Build history of the part. All positions in model axes, mm. Give positions to 0.01 mm unless a question says otherwise; leave off trailing zeros. Order: outer loops, then holes, each group sorted by start corner. A loop starts at its lowest first (then second) coordinate and runs counter-clockwise, first axis right, second up. Notation, with made-up numbers: (14.5, 36) - (20.5, 36) arc R22 ccw to (20.5, 45) - close; hole circle Ø10 at (-21.5, 48). An arc over 180 degrees is marked (long way). One line per item, written item: value.
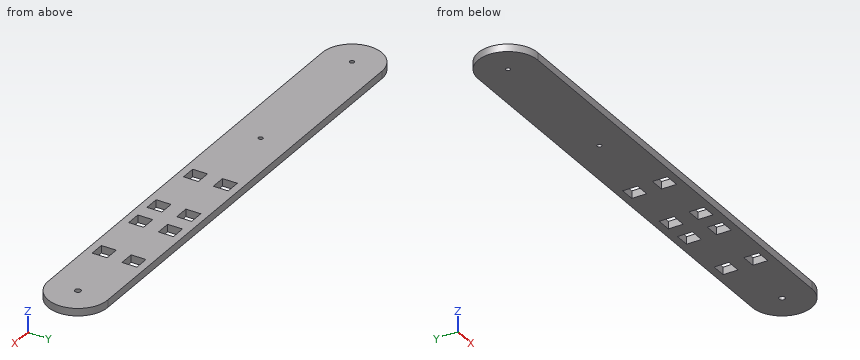
```python
from build123d import *

# Parameters (mm, degrees)
SKETCH1_R           = 1.5
SKETCH1_R_2         = 2
SKETCH1_W           = 10
SKETCH1_H           = 10
BOSS_EXTRUDE1_DEPTH = 5


with BuildPart() as part:
    # Sketch1 → Boss-Extrude1 (new body)
    with BuildSketch(Plane.XY):
        with BuildLine():
            Line((-126.904376013, 20), (173.095623987, 20))
            ThreePointArc((173.095623987, 20), (193.095623987, 0), (173.095623987, -20))
            Line((173.095623987, -20), (-126.904376013, -20))
            ThreePointArc((-126.904376013, -20), (-146.904376013, 0), (-126.904376013, 20))
        make_face()
        with Locations((-126.904376013, 0)):
            Circle(SKETCH1_R, mode=Mode.SUBTRACT)
        with Locations((173.095623987, 0)):
            Circle(SKETCH1_R_2, mode=Mode.SUBTRACT)
        with Locations((-26.904376013, 0)):
            Circle(SKETCH1_R, mode=Mode.SUBTRACT)
        Polygon((63.095623987, 15), (73.095623987, 15), (73.095623987, 10), (73.095623987, 5), (63.095623987, 5), (63.095623987, 10), align=None, mode=Mode.SUBTRACT)
        Polygon((83.095623987, 10), (83.095623987, 5), (93.095623987, 5), (93.095623987, 10), (93.095623987, 15), (83.095623987, 15), align=None, mode=Mode.SUBTRACT)
        Polygon((123.095623987, 10), (123.095623987, 5), (133.095623987, 5), (133.095623987, 10), (133.095623987, 15), (123.095623987, 15), align=None, mode=Mode.SUBTRACT)
        Polygon((33.095623987, -15), (23.095623987, -15), (23.095623987, -10), (23.095623987, -5), (33.095623987, -5), (33.095623987, -10), align=None, mode=Mode.SUBTRACT)
        Polygon((63.095623987, -15), (73.095623987, -15), (73.095623987, -10), (73.095623987, -5), (63.095623987, -5), (63.095623987, -10), align=None, mode=Mode.SUBTRACT)
        Polygon((83.095623987, -10), (83.095623987, -5), (93.095623987, -5), (93.095623987, -10), (93.095623987, -15), (83.095623987, -15), align=None, mode=Mode.SUBTRACT)
        Polygon((123.095623987, -5), (133.095623987, -5), (133.095623987, -10), (133.095623987, -15), (123.095623987, -15), (123.095623987, -10), align=None, mode=Mode.SUBTRACT)
        with Locations((28.095623987, 10)):
            Rectangle(SKETCH1_W, SKETCH1_H, mode=Mode.SUBTRACT)
    extrude(amount=BOSS_EXTRUDE1_DEPTH)


solid = part.part
```
(1) Pin check, flat tips, straight feed: P1, Ø2.5, axis at y = -9.5, z = 3, coming from the +X side; P2, Ø1.5, axis at y = 11, z = 3.5, coming from the -X side; P3, Ø1.5, axis at y = 11, z = 2.5, coming from the +X side. Stop position of each tip, or through.
Completed:
P1: x = 191.31
P2: x = -144.08
P3: x = 190.27
(2) Drill centre lines: line 1 (Y direction, x = 86, z = 2); line 2 (X direction, y = 14.5, z = 0.3); line 3 (X direction, y = -0.5, z = 1.25). Where is each one in solid material? Low to high.
Completed:
line 1: -20 to -15, -5 to 5, 15 to 20
line 2: -140.68 to 23.1, 33.1 to 63.1, 73.1 to 83.1, 93.1 to 123.1, 133.1 to 186.87
line 3: -146.9 to -128.32, -125.49 to -28.32, -25.49 to 171.16, 175.03 to 193.09
(3) Slice it at B-B, the plane z = 3. Count the separate pieces of the cut face and the enclosed holes in it, and give its area (3 significant figures).
Completed:
separate pieces: 1
enclosed holes: 11
area: 12,400 mm²
(4) Slice it at A-A, the plane y = -8.5. Give the cut face in (x, z).
Completed:
outline: (-145.01, 0) - (23.1, 0) - (23.1, 5) - (-145.01, 5) - close; (33.1, 0) - (63.1, 0) - (63.1, 5) - (33.1, 5) - close; (73.1, 0) - (83.1, 0) - (83.1, 5) - (73.1, 5) - close; (93.1, 0) - (123.1, 0) - (123.1, 5) - (93.1, 5) - close; (133.1, 0) - (191.2, 0) - (191.2, 5) - (133.1, 5) - close
